```python
from build123d import *

# Parameters (mm, degrees)
BOSS_EXTRUDE1_DEPTH = 24
SKETCH4_R           = 6.5
BOSS_EXTRUDE2_DEPTH = 24
SKETCH3_R           = 3
CUT_EXTRUDE1_DEPTH  = 30.899298428
FILLET1_R           = 3
CHAMFER1_SIZE       = 1


with BuildPart() as part:
    # Sketch1 → Boss-Extrude1 (new body)
    with BuildSketch(Plane.XY):
        Polygon((0, 15), (14.899298428, 15), (14.899298428, -14.949649214), (-15, -14.949649214), (-15, 15), align=None)
        Polygon((-10, 10), (-4.792538857, 10), (-3.1, 8.307461143), (-5.5, 8.307461143), (-5.5, 6.667461143), (-2.79, 3.957461143), (2.79, 3.957461143), (5.5, 6.667461143), (5.5, 8.307461143), (3.1, 8.307461143), (4.792538857, 10), (10, 10), (10, 4.792538857), (8.307461143, 3.1), (8.307461143, 5.5), (6.667461143, 5.5), (3.957461143, 2.79), (3.957461143, -2.79), (6.667461143, -5.5), (8.307461143, -5.5), (8.307461143, -3.1), (10, -4.792538857), (10, -10), (4.792538857, -10), (3.1, -8.307461143), (5.5, -8.307461143), (5.5, -6.667461143), (2.79, -3.957461143), (-2.79, -3.957461143), (-5.5, -6.667461143), (-5.5, -8.307461143), (-3.1, -8.307461143), (-4.792538857, -10), (-10, -10), (-10, -4.792538857), (-8.307461143, -3.1), (-8.307461143, -5.5), (-6.667461143, -5.5), (-3.957461143, -2.79), (-3.957461143, 2.79), (-6.667461143, 5.5), (-8.307461143, 5.5), (-8.307461143, 3.1), (-10, 4.792538857), align=None, mode=Mode.SUBTRACT)
    extrude(amount=BOSS_EXTRUDE1_DEPTH)

    # Sketch4 → Boss-Extrude2 (add)
    with BuildSketch(Plane(origin=(0, 0, 0), x_dir=(-1, 0, 0), z_dir=(0, 0, -1))):
        with BuildLine():
            ThreePointArc((-14.899298428, 26.5), (0.050350786, 41.449649214), (15, 26.5))
            Line((15, 26.5), (15, 15))
            Line((15, 15), (-14.899298428, 15))
            Line((-14.899298428, 15), (-14.899298428, 26.5))
        make_face()
        with Locations((0.050350786, 26.5)):
            Circle(SKETCH4_R, mode=Mode.SUBTRACT)
    extrude(amount=-BOSS_EXTRUDE2_DEPTH)

    # Sketch3 → Cut-Extrude1 (cut, through all)
    with BuildSketch(Plane.ZY.offset(15)):
        with Locations((12, 0)):
            Circle(SKETCH3_R)
    extrude(amount=-CUT_EXTRUDE1_DEPTH, mode=Mode.SUBTRACT)

    # Fillet1
    fillet1_edges = [part.edges().sort_by_distance(p)[0] for p in [
        (-0.050350786, -14.949649214, 24),
        (14.899298428, 5.775175393, 24),
        (-0.050350786, 41.449649214, 24),
        (-0.050350786, 41.449649214, 0),
        (14.899298428, 5.775175393, 0),
        (-0.050350786, -14.949649214, 0),
        (-15, 5.775175393, 0),
        (-15, 5.775175393, 24),
        (14.899298428, -14.949649214, 12),
        (-15, -14.949649214, 12),
    ]]
    fillet(fillet1_edges, radius=FILLET1_R)

    # Chamfer1
    chamfer1_edges = [part.edges().sort_by_distance(p)[0] for p in [
        (6.449649214, 26.5, 24),
        (6.449649214, 26.5, 0),
        (-4.3, 8.307461143, 0),
        (-3.946269429, 9.153730571, 0),
        (-7.396269429, 10, 0),
        (-10, 7.396269429, 0),
        (-9.153730571, 3.946269429, 0),
        (-8.307461143, 4.3, 0),
        (-7.487461143, 5.5, 0),
        (-5.312461143, 4.145, 0),
        (-3.957461143, 0, 0),
        (-5.312461143, -4.145, 0),
        (-7.487461143, -5.5, 0),
        (-8.307461143, -4.3, 0),
        (-9.153730571, -3.946269429, 0),
        (-10, -7.396269429, 0),
        (-7.396269429, -10, 0),
        (-3.946269429, -9.153730571, 0),
        (-4.3, -8.307461143, 0),
        (-5.5, -7.487461143, 0),
        (-4.145, -5.312461143, 0),
        (0, -3.957461143, 0),
        (4.145, -5.312461143, 0),
        (5.5, -7.487461143, 0),
        (4.3, -8.307461143, 0),
        (3.946269429, -9.153730571, 0),
        (7.396269429, -10, 0),
        (10, -7.396269429, 0),
        (9.153730571, -3.946269429, 0),
        (8.307461143, -4.3, 0),
        (7.487461143, -5.5, 0),
        (5.312461143, -4.145, 0),
        (3.957461143, 0, 0),
        (5.312461143, 4.145, 0),
        (7.487461143, 5.5, 0),
        (8.307461143, 4.3, 0),
        (9.153730571, 3.946269429, 0),
        (10, 7.396269429, 0),
        (7.396269429, 10, 0),
        (3.946269429, 9.153730571, 0),
        (4.3, 8.307461143, 0),
        (5.5, 7.487461143, 0),
        (4.145, 5.312461143, 0),
        (0, 3.957461143, 0),
        (-4.145, 5.312461143, 0),
        (-5.5, 7.487461143, 0),
        (-4.3, 8.307461143, 24),
        (-3.946269429, 9.153730571, 24),
        (-7.396269429, 10, 24),
        (-10, 7.396269429, 24),
        (-9.153730571, 3.946269429, 24),
        (-8.307461143, 4.3, 24),
        (-7.487461143, 5.5, 24),
        (-5.312461143, 4.145, 24),
        (-3.957461143, 0, 24),
        (-5.312461143, -4.145, 24),
        (-7.487461143, -5.5, 24),
        (-8.307461143, -4.3, 24),
        (-9.153730571, -3.946269429, 24),
        (-10, -7.396269429, 24),
        (-7.396269429, -10, 24),
        (-3.946269429, -9.153730571, 24),
        (-4.3, -8.307461143, 24),
        (-5.5, -7.487461143, 24),
        (-4.145, -5.312461143, 24),
        (0, -3.957461143, 24),
        (4.145, -5.312461143, 24),
        (5.5, -7.487461143, 24),
        (4.3, -8.307461143, 24),
        (3.946269429, -9.153730571, 24),
        (7.396269429, -10, 24),
        (10, -7.396269429, 24),
        (9.153730571, -3.946269429, 24),
        (8.307461143, -4.3, 24),
        (7.487461143, -5.5, 24),
        (5.312461143, -4.145, 24),
        (3.957461143, 0, 24),
        (5.312461143, 4.145, 24),
        (7.487461143, 5.5, 24),
        (8.307461143, 4.3, 24),
        (9.153730571, 3.946269429, 24),
        (10, 7.396269429, 24),
        (7.396269429, 10, 24),
        (3.946269429, 9.153730571, 24),
        (4.3, 8.307461143, 24),
        (5.5, 7.487461143, 24),
        (4.145, 5.312461143, 24),
        (0, 3.957461143, 24),
        (-4.145, 5.312461143, 24),
        (-5.5, 7.487461143, 24),
    ]]
    chamfer(chamfer1_edges, length=CHAMFER1_SIZE)


solid = part.part
```
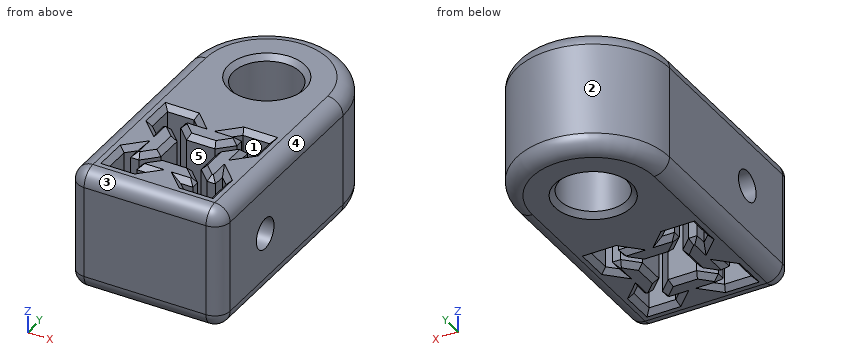
The model under review builds one solid part; all positions refer to its coordinate system, in mm. Face numbers are marked on the shaded views. A direction names the side the tool comes from. Round coordinates to 2 decimals unless told otherwise and drop trailing zeros. Loops run counter-clockwise (first coordinate to the right, second up) from the corner with the lowest first, then second, coordinate; pieces in that order, holes last. Notation, with made-up numbers: M 52,15 L 69,15 A11 ccw 69,20 Z; hole C 27,38 d11. An arc over 180 degrees is marked long. Write item = value, one per line.
Item 1: Take a section at B-B on z = 12.25. State how many separate pieces and enclosed holes the cut face has, then the cut area to 3 significant figures.
Return value:
separate_pieces = 2
enclosed_holes = 1
area = 1,140 mm2
Item 2: The part is to be moulded in two halves that separate along X. For the marked faces 1, 2 and 3, say which applies: released by +X, released by -X, zero draft, split by the parting line, or undercut.
Return value:
face_1 = undercut
face_2 = split by the parting line
face_3 = zero draft
Item 3: Take a section at A-A on y = 0. Write out the cut boundary in (x, z).
Return value:
outline = M -15,3 A3 ccw -12,0 L -4.96,0 L -3.96,1 L -3.96,9 L -15,9 Z; M -15,15 L -3.96,15 L -3.96,23 L -4.96,24 L -12,24 A3 ccw -15,21 Z; M 3.96,1 L 4.96,0 L 11.9,0 A3 ccw 14.9,3 L 14.9,9 L 3.96,9 Z; M 3.96,15 L 14.9,15 L 14.9,21 A3 ccw 11.9,24 L 4.96,24 L 3.96,23 Z
Item 4: Machinability: for the marked faces 4 and 5, which of the approach directions +Z, -Z, +X, -X, +Y, -Y give a long, thin tool a straight path to every point of the face, cutting with its end or side? Answer none if there is none.
Return value:
face_4 = +Z, +X, +Y, -Y
face_5 = +Z, -Z
Item 5: Insertion check: P1, Ø1.7, axis at x = -1, z = 7, coming from the +Y side; P2, Ø3, axis at x = 5, z = 11.5, coming from the +Y side; P3, Ø10, axis at x = -12, z = 11, coming from the +Y side; P4, Ø3, axis at x = -9.5, z = 3, coming from the +Y side. Each pin has a flat end and moves straight along its axis. Give the tip position at first contact, or say it passes through.
Return value:
P1 = 41.45
P2 = 41.02
P3 = 39.74
P4 = 39.16
Item 6: For line 1 (Y direction, x = 0, z = 17.75); line 2 (X direction, y = 7.5, z = 6); line 3 (Z direction, x = 11.25, y = 0), list the stretches that pass through material, from the lowest coordinate up. Write a range as [from, to].
Return value:
line_1 = [-14.95, -3.96], [3.96, 20], [33, 41.45]
line_2 = [-15, -10], [-5.5, 5.5], [10, 14.9]
line_3 = [0, 9], [15, 24]
